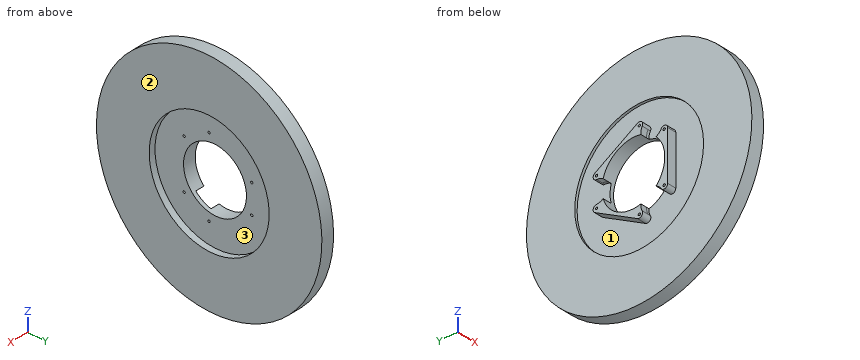
from build123d import *

# Parameters (mm, degrees)
SKETCH1_R                   = 89.825
SKETCH1_R_2                 = 47.825
BOSS_EXTRUDE1_DEPTH         = 10
SKETCH3_R                   = 47.825
TBH_IDK_DEPTH               = 5
EXTRUSION_START             = 5
SKETCH4_R                   = 47.825
EXTRUSION_TO_FUEL_MAN_DEPTH = 5
OX_DOWNCOMER_REACH          = 129.914
OX_PROFILE_R                = 0.914623685
OX_ORIFICES_COUNT           = 3
SKETCH7_R                   = 47.825
FUEL_BLOCKERS_DEPTH         = 5
SKETCH8_R                   = 25.085
TI_CUT_EXTRUDE_DEPTH        = 128.424727781
SKETCH9_R                   = 51.325
FUEL_VOLUME_DEPTH           = 2


with BuildPart() as part:
    # Sketch1 → Boss-Extrude1 (new body)
    with BuildSketch(Plane(origin=(0, 0, 0), x_dir=(0, 0, -1), z_dir=(1, 0, 0))):
        Circle(SKETCH1_R)
        Circle(SKETCH1_R_2, mode=Mode.SUBTRACT)
    extrude(amount=BOSS_EXTRUDE1_DEPTH)

    # Sketch3 → tbh idk (add)
    with BuildSketch(Plane.ZY):
        Circle(SKETCH3_R)
    extrude(amount=-TBH_IDK_DEPTH)

    # Sketch4 → Extrusion to Fuel Man (add)
    with BuildSketch(Plane.ZY.offset(EXTRUSION_START)):
        Circle(SKETCH4_R)
    extrude(amount=-EXTRUSION_TO_FUEL_MAN_DEPTH)

    # Ox Profile → Ox Downcomer (cut, up to next)
    with BuildSketch(Plane.ZY.offset(5), mode=Mode.PRIVATE) as ox_downcomer_sk1:
        with Locations((11.464101615, 29.2826)):
            Circle(OX_PROFILE_R)
    ox_downcomer_tool1 = extrude(ox_downcomer_sk1.sketch, amount=-OX_DOWNCOMER_REACH, mode=Mode.PRIVATE) & part.part
    # Ox Profile → Ox Downcomer (cut, up to next)
    with BuildSketch(Plane.ZY.offset(5), mode=Mode.PRIVATE) as ox_downcomer_sk2:
        with Locations((-11.464101615, 29.2826)):
            Circle(OX_PROFILE_R)
    ox_downcomer_tool2 = extrude(ox_downcomer_sk2.sketch, amount=-OX_DOWNCOMER_REACH, mode=Mode.PRIVATE) & part.part
    ox_downcomer_1 = ox_downcomer_tool1.solids().sort_by_distance((-5, 29.2826, 11.464102))[0]
    add(ox_downcomer_1, mode=Mode.SUBTRACT)
    ox_downcomer_2 = ox_downcomer_tool2.solids().sort_by_distance((-5, 29.2826, -11.464102))[0]
    add(ox_downcomer_2, mode=Mode.SUBTRACT)
    ox_downcomer = ox_downcomer_1 + ox_downcomer_2  # Ox Downcomer as one shape, for the pattern or mirror that repeats it

    # Ox Orifices: Ox Downcomer ×3 about axis
    ox_orifices_axis = Axis((0, -0.021435438, 0), (1, 0, 0))
    for i in range(1, OX_ORIFICES_COUNT):
        add(ox_downcomer.rotate(ox_orifices_axis, i * 360 / OX_ORIFICES_COUNT), mode=Mode.SUBTRACT)

    # Sketch7 → Fuel Blockers (cut)
    with BuildSketch(Plane.ZY.offset(5)):
        Circle(SKETCH7_R)
        with BuildLine():
            Line((-33.467788335, -3.341161242), (-13.840363653, 30.654535527))
            ThreePointArc((-13.840363653, 30.654535527), (-10.753935529, 31.932975916), (-8.72023056, 29.2826))
            ThreePointArc((-8.72023056, 29.2826), (0, 20.56236944), (8.72023056, 29.2826))
            ThreePointArc((8.72023056, 29.2826), (10.753935529, 31.932975916), (13.840363653, 30.654535527))
            Line((13.840363653, 30.654535527), (33.467788335, -3.341161242))
            ThreePointArc((33.467788335, -3.341161242), (33.031736126, -6.653306599), (29.719590769, -7.089358808))
            ThreePointArc((29.719590769, -7.089358808), (17.807534297, -10.28118472), (20.999360209, -22.193241192))
            ThreePointArc((20.999360209, -22.193241192), (22.277800597, -25.279669317), (19.627424681, -27.313374285))
            Line((19.627424681, -27.313374285), (-19.627424681, -27.313374285))
            ThreePointArc((-19.627424681, -27.313374285), (-22.277800597, -25.279669317), (-20.999360209, -22.193241192))
            ThreePointArc((-20.999360209, -22.193241192), (-17.807534297, -10.28118472), (-29.719590769, -7.089358808))
            ThreePointArc((-29.719590769, -7.089358808), (-33.031736126, -6.653306599), (-33.467788335, -3.341161242))
        make_face(mode=Mode.SUBTRACT)
    extrude(amount=-FUEL_BLOCKERS_DEPTH, mode=Mode.SUBTRACT)

    # Sketch8 → TI Cut Extrude (cut, through all)
    with BuildSketch(Plane(origin=(5, 0, 0), x_dir=(0, 0, -1), z_dir=(1, 0, 0))):
        Circle(SKETCH8_R)
    extrude(amount=-TI_CUT_EXTRUDE_DEPTH, mode=Mode.SUBTRACT)

    # Sketch9 → Fuel Volume (cut)
    with BuildSketch(Plane.ZY):
        Circle(SKETCH9_R)
        with BuildLine():
            ThreePointArc((-13.840363653, 30.654535527), (-10.753935529, 31.932975916), (-8.72023056, 29.2826))
            ThreePointArc((-8.72023056, 29.2826), (-8.280001273, 26.546909971), (-7.003762198, 24.087435315))
            ThreePointArc((-7.003762198, 24.087435315), (0, 25.085), (7.003762198, 24.087435315))
            ThreePointArc((7.003762198, 24.087435315), (8.280001273, 26.546909971), (8.72023056, 29.2826))
            ThreePointArc((8.72023056, 29.2826), (10.753935529, 31.932975916), (13.840363653, 30.654535527))
            Line((13.840363653, 30.654535527), (33.467788335, -3.341161242))
            ThreePointArc((33.467788335, -3.341161242), (33.031736126, -6.653306599), (29.719590769, -7.089358808))
            ThreePointArc((29.719590769, -7.089358808), (27.130299064, -6.102763539), (24.362211994, -5.978281672))
            ThreePointArc((24.362211994, -5.978281672), (21.724247254, -12.5425), (17.358449796, -18.109153643))
            ThreePointArc((17.358449796, -18.109153643), (18.85029779, -20.444146432), (20.999360209, -22.193241192))
            ThreePointArc((20.999360209, -22.193241192), (22.277800597, -25.279669317), (19.627424681, -27.313374285))
            Line((19.627424681, -27.313374285), (-19.627424681, -27.313374285))
            ThreePointArc((-19.627424681, -27.313374285), (-22.277800597, -25.279669317), (-20.999360209, -22.193241192))
            ThreePointArc((-20.999360209, -22.193241192), (-18.85029779, -20.444146432), (-17.358449796, -18.109153643))
            ThreePointArc((-17.358449796, -18.109153643), (-21.724247254, -12.5425), (-24.362211994, -5.978281672))
            ThreePointArc((-24.362211994, -5.978281672), (-27.130299064, -6.102763539), (-29.719590769, -7.089358808))
            ThreePointArc((-29.719590769, -7.089358808), (-33.031736126, -6.653306599), (-33.467788335, -3.341161242))
            Line((-33.467788335, -3.341161242), (-13.840363653, 30.654535527))
        make_face(mode=Mode.SUBTRACT)
    extrude(amount=-FUEL_VOLUME_DEPTH, mode=Mode.SUBTRACT)


solid = part.part
The model under review builds one solid part; all positions refer to its coordinate system, in mm. Face numbers are marked on the shaded views. Round coordinates to 2 decimals unless told otherwise and drop trailing zeros. Loops run counter-clockwise (first coordinate to the right, second up) from the corner with the lowest first, then second, coordinate; pieces in that order, holes last. Notation, with made-up numbers: (42.5, 75) -> (71.5, 75) arc R19 ccw to (71.5, 95) -> close; hole circle Ø5 at (-24.5, 69.25). An arc over 180 degrees is marked (long way). Return JSON: item names as keys, results as strings.
(1) Add section C-C on z = 0. Write out the cut boundary in (x, y) (3 decimals).
Solved:
{"outline": "(-5, -27.313) -> (2, -27.313) -> (2, -51.325) -> (0, -51.325) -> (0, -89.825) -> (10, -89.825) -> (10, -47.825) -> (5, -47.825) -> (5, -25.085) -> (-5, -25.085) -> close; (0, 51.325) -> (2, 51.325) -> (2, 25.085) -> (5, 25.085) -> (5, 47.825) -> (10, 47.825) -> (10, 89.825) -> (0, 89.825) -> close"}
(2) Add section A-A on x = -2.5. State how many separate pieces and enclosed holes the cut face has, plus the area to 3 significant figures.
Solved:
{"separate pieces": "3", "enclosed holes": "6", "area": "617 mm2"}
(3) For pin 1 (2 mm diameter, centred on y = 29.28, z = 11.46, fed in from +X); pin 2 (3 mm diameter, centred on x = 6, z = 23.5, fed in from +Y); pin 3 (8 mm diameter, centred on x = 6, z = -20, fed in from +Y), all flat-tipped, find the tip position at first contact; note any pin that passes through.
Solved:
{"pin 1": "x = 5", "pin 2": "y = 87.09", "pin 3": "y = 88.39"}
(4) The part is to be moulded in two halves that separate along Z. For the marked faces 1, 2 and 3, say which applies: released by +Z, released by -Z, zero draft, split by the parting line, or undercut.
Solved:
{"face 1": "undercut", "face 2": "zero draft", "face 3": "undercut"}
(5) For line 1 (Z direction, x = 1.75, y = 6); line 2 (Y direction, x = -1.75, z = 12); line 3 (X direction, y = 11.5, z = -31.5), list the stretches that pass through material, from the lowest coordinate up.
Solved:
{"line 1": "-89.62 to -50.97, -28.07 to -24.36, 24.36 to 28.07, 50.97 to 89.62", "line 2": "-27.31 to -22.03, 22.03 to 28.54, 30.02 to 31.97", "line 3": "2 to 5"}
(6) Add section D-D on z = -45. Write out the cut boundary in (x, y), plus the area to 3 significant figures.
Solved:
{"outline": "(0, -77.74) -> (10, -77.74) -> (10, -16.19) -> (5, -16.19) -> (5, 16.19) -> (10, 16.19) -> (10, 77.74) -> (0, 77.74) -> (0, 24.68) -> (2, 24.68) -> (2, -24.68) -> (0, -24.68) -> close", "area": "1,290 mm2"}
(7) Add section B-B on y = 15.5. Write out the cut boundary in (x, z).
Solved:
{"outline": "(-5, -22.59) -> (2, -22.59) -> (2, -48.93) -> (0, -48.93) -> (0, -88.48) -> (10, -88.48) -> (10, -45.24) -> (5, -45.24) -> (5, -19.72) -> (-5, -19.72) -> close; (-5, 19.72) -> (5, 19.72) -> (5, 45.24) -> (10, 45.24) -> (10, 88.48) -> (0, 88.48) -> (0, 48.93) -> (2, 48.93) -> (2, 22.59) -> (-5, 22.59) -> close"}
